```python
from build123d import *

# Parameters (mm, degrees)
SKETCH2_R           = 20
BOSS_EXTRUDE1_DEPTH = 220
SKETCH3_W           = 30
SKETCH3_H           = 41.781255482
CUT_EXTRUDE1_DEPTH  = 25
SKETCH4_R           = 2.5
CUT_EXTRUDE2_DEPTH  = 2.5


with BuildPart() as part:
    # Sketch2 → Boss-Extrude1 (new body)
    with BuildSketch(Plane(origin=(0, 0, 0), x_dir=(1, 0, 0), z_dir=(0, 1, 0))):
        Circle(SKETCH2_R)
    extrude(amount=BOSS_EXTRUDE1_DEPTH)

    # Sketch3 → Cut-Extrude1 (cut)
    with BuildSketch(Plane(origin=(0, 220, 0), x_dir=(1, 0, 0), z_dir=(0, 1, 0))):
        Rectangle(SKETCH3_W, SKETCH3_H)
    extrude(amount=-CUT_EXTRUDE1_DEPTH, mode=Mode.SUBTRACT)

    # Sketch4 → Cut-Extrude2 (cut)
    with BuildSketch(Plane(origin=(-15, 0, 0), x_dir=(0, 0, -1), z_dir=(1, 0, 0))):
        with Locations((0, 215)):
            Circle(SKETCH4_R)
    cut_extrude2 = extrude(amount=-CUT_EXTRUDE2_DEPTH, mode=Mode.SUBTRACT)

    # Mirror1: Cut-Extrude2 across plane
    add(cut_extrude2.mirror(Plane(origin=(0, 0, 0), x_dir=(0, 0, 1), z_dir=(1, 0, 0))), mode=Mode.SUBTRACT)


solid = part.part
```
Input: part model. Units: mm. Frame: model coordinates. A direction names the side the tool comes from. Coordinates: 2 decimals unless noted, no trailing zeros. Write each loop counter-clockwise with the first axis right and the second up, starting at its lowest first coordinate (ties: lowest second). Pieces come first, ordered by that corner, then holes.
1) Set-up query: faces 1 (the flat face through (15, 208, 0)), 2 (the cylindrical face through (16.23, 217.48, 0.33)), 3 (the flat face through (-17, 220, 0)). Return all of +Z, -Z, +X, -X, +Y, -Y with unobstructed straight access to the full face (end or side cutting, diameter ignored); none if empty.
2) Section C-C on x = 0. Output: boundary loops of the cut face in (y, z).
3) Mould query, pull axis Y, two halves, no side actions, for faces 4 (the cylindrical face through (-4.336, 108.46, 19.524)), 5 (the flat face through (0, 195, 0)), 6 (the flat face through (17.5, 215, 0)). Classes: pulls with the +Y half, pulls with the -Y half, needs draft (parallel to the pull), parting line crosses it, or undercut.
4) Section D-D on y = 143. Output: boundary loops of the cut face in (x, z).
5) Section A-A on y = 215. Output: boundary loops of the cut face in (x, z), and give its area (3 significant figures).
6) Section B-B on z = 0. Output: boundary loops of the cut face in (x, y).
7) Pin query (flat end, axial travel): pin 1 Ø12 at (y, z) = (136, -7.5) entering from +X; pin 2 Ø1 at (y, z) = (168.5, 13.5) entering from +X; pin 3 Ø10 at (y, z) = (87.5, -14) entering from -X. Return the tip coordinate at first contact, or that it passes through.
8) Material intervals for line 1 along Y through (x, z) = (16, 0); line 2 along Y through (x, z) = (4.5, 9); line 3 along Z through (x, y) = (0.5, 108), sorted ascending.
Check result:
1. face 1: +Z, -Z, +Y
1. face 2: none
1. face 3: +Z, -Z, +X, -X, +Y
2. outline: (0, -20) - (195, -20) - (195, 20) - (0, 20) - close
3. face 4: needs draft
3. face 5: pulls with the +Y half
3. face 6: undercut
4. outline: circle Ø40 at (0, 0)
5. outline: (-17.5, -2.5) - (-17.5, 2.5) - (-15, 2.5) - (-15, 13.23) arc R20 ccw to (-15, -13.23) - (-15, -2.5) - close; (15, -13.23) arc R20 ccw to (15, 13.23) - (15, 2.5) - (17.5, 2.5) - (17.5, -2.5) - (15, -2.5) - close
5. area: 156 mm2
6. outline: (-20, 0) - (20, 0) - (20, 220) - (15, 220) - (15, 217.5) - (17.5, 217.5) - (17.5, 212.5) - (15, 212.5) - (15, 195) - (-15, 195) - (-15, 212.5) - (-17.5, 212.5) - (-17.5, 217.5) - (-15, 217.5) - (-15, 220) - (-20, 220) - close
7. pin 1: stops at x = 19.94
7. pin 2: stops at x = 15.2
7. pin 3: stops at x = -17.86
8. line 1: y = 0 to 212.5, 217.5 to 220
8. line 2: y = 0 to 195
8. line 3: z = -19.99 to 19.99
